from build123d import *

# Parameters (mm, degrees)
SKETCH1_W                                   = 37
SKETCH1_H                                   = 61
BASE_EXTRUSION_DEPTH                        = 1.5875
M2_CLEARANCE_HOLE3_D                        = 2.2
SKETCH8_W                                   = 0.5
SKETCH8_H                                   = 2.2
SIDE_SLOTS_DEPTH                            = 36.707424386
CORNER_BOSS_CLEARANCE_DEPTH                 = 36.707424386
CORNER_BOSS_CLEARANCE_MIRROR_2_COPY_1_DEPTH = 36.707424386
SKETCH10_R                                  = 1.1
AC_WIRE_HOLES_DEPTH                         = 36.707424386


with BuildPart() as part:
    # Sketch1 → Base Extrusion (new body)
    with BuildSketch(Plane(origin=(0, 0, 0), x_dir=(1, 0, 0), z_dir=(0, 1, 0))):
        Rectangle(SKETCH1_W, SKETCH1_H)
    extrude(amount=BASE_EXTRUSION_DEPTH)

    # M2 Clearance Hole3 (through all)
    with Locations(Plane(origin=(0, 1.5875, 0), x_dir=(1, 0, 0), z_dir=(0, 1, 0))):
        with Locations((-18, 10), (-18, -10), (18, -10), (18, 10)):
            Hole(M2_CLEARANCE_HOLE3_D / 2)

    # Sketch8 → Side Slots (cut, through all)
    with BuildSketch(Plane(origin=(0, 1.5875, 0), x_dir=(1, 0, 0), z_dir=(0, 1, 0))):
        with Locations((-18.25, 10)):
            Rectangle(SKETCH8_W, SKETCH8_H)
        with Locations((-18.25, -10)):
            Rectangle(SKETCH8_W, SKETCH8_H)
        with Locations((18.25, 10)):
            Rectangle(SKETCH8_W, SKETCH8_H)
        with Locations((18.25, -10)):
            Rectangle(SKETCH8_W, SKETCH8_H)
    extrude(amount=-SIDE_SLOTS_DEPTH, mode=Mode.SUBTRACT)

    # Sketch9 → Corner Boss Clearance (cut, through all)
    with BuildSketch(Plane(origin=(0, 1.5875, 0), x_dir=(1, 0, 0), z_dir=(0, 1, 0))):
        with BuildLine():
            Line((-18.5, -32.8), (-10.5, -32.8))
            Line((-10.5, -32.8), (-10.5, -28.8))
            ThreePointArc((-10.5, -28.8), (-11.671572875, -25.971572875), (-14.5, -24.8))
            Line((-14.5, -24.8), (-18.5, -24.8))
            Line((-18.5, -24.8), (-18.5, -32.8))
        make_face()
    corner_boss_clearance = extrude(amount=-CORNER_BOSS_CLEARANCE_DEPTH, mode=Mode.SUBTRACT)

    # Corner Boss Clearance Mirror: Corner Boss Clearance across plane
    add(corner_boss_clearance.mirror(Plane(origin=(0, 0, 0), x_dir=(0, 0, 1), z_dir=(1, 0, 0))), mode=Mode.SUBTRACT)

    # Corner Boss Clearance Mirror 2: Corner Boss Clearance across plane
    add(corner_boss_clearance.mirror(Plane.XY), mode=Mode.SUBTRACT)

    # Corner Boss Clearance Mirror 2 copy 1 sk → Corner Boss Clearance Mirror 2 copy 1 (cut, through all)
    with BuildSketch(Plane(origin=(0, 1.5875, 0), x_dir=(-1, 0, 0), z_dir=(0, 1, 0))):
        with BuildLine():
            Line((-18.5, -32.8), (-10.5, -32.8))
            Line((-10.5, -32.8), (-10.5, -28.8))
            ThreePointArc((-10.5, -28.8), (-11.671572875, -25.971572875), (-14.5, -24.8))
            Line((-14.5, -24.8), (-18.5, -24.8))
            Line((-18.5, -24.8), (-18.5, -32.8))
        make_face()
    extrude(amount=-CORNER_BOSS_CLEARANCE_MIRROR_2_COPY_1_DEPTH, mode=Mode.SUBTRACT)

    # Sketch10 → AC Wire Holes (cut, through all)
    with BuildSketch(Plane.XZ):
        with Locations(Location((-5, -27.4, 0), (0, 0, 270))):
            Circle(SKETCH10_R)
        with Locations(Location((5, -27.4, 0), (0, 0, 270))):
            Circle(SKETCH10_R)
        with Locations(Location((-15.4, 17.95, 0), (0, 0, 270))):
            Circle(SKETCH10_R)
        with Locations(Location((-15.4, 2.05, 0), (0, 0, 270))):
            Circle(SKETCH10_R)
    extrude(amount=-AC_WIRE_HOLES_DEPTH, mode=Mode.SUBTRACT)


solid = part.part
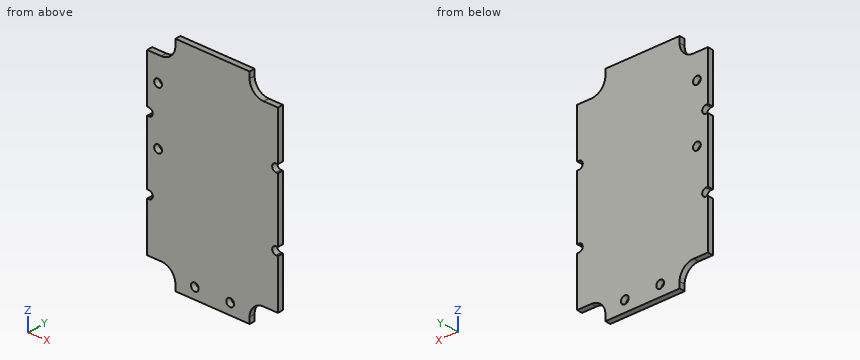
Geometry check sheet. Reference: the model listing, model coordinates, mm. Round coordinates to 2 decimals unless told otherwise and drop trailing zeros. Loops run counter-clockwise (first coordinate to the right, second up) from the corner with the lowest first, then second, coordinate; pieces in that order, holes last. Notation, with made-up numbers: (-14, 43.5) -> (35, 43.5) arc R33 cw to (35, 75.5) -> close; hole circle Ø6 at (67.5, 54). An arc over 180 degrees is marked (long way). Answer as a JSON object with one key per item and string values. Group by question number.
Item 1: Depth check by flat-ended pin: pin 1 Ø0.8 at (y, z) = (1, -30) entering from +X; pin 2 Ø0.5 at (y, z) = (0.5, -29.5) entering from -X. Enter the tip coordinate at first touch or a pass-through.
Item 2: Cross-section at A-A, the plane x = -15.4. Record the cut outline in (y, z).
Item 3: Thickness scan on line 1 along X through (y, z) = (0.5, -27.4); line 2 along X through (y, z) = (0.55, 2.05); line 3 along Z through (x, y) = (-5.5, 0.55). Record the ranges inside material, lowest first.
Item 4: Cross-section at C-C, the plane x = 5. Record the cut outline in (y, z), plus the area to 3 significant figures.
Item 5: Cross-section at B-B, the plane z = 17.95. Record the cut outline in (x, y).
Item 6: Cross-section at D-D, the plane z = -27.4. Record the cut outline in (x, y), plus the area to 3 significant figures.
Determined:
{
 "1": {"pin 1": "stops at x = 10.5", "pin 2": "stops at x = -10.5"},
 "2": {"outline": "(0, -24.8) -> (1.59, -24.8) -> (1.59, 0.95) -> (0, 0.95) -> close; (0, 3.15) -> (1.59, 3.15) -> (1.59, 16.85) -> (0, 16.85) -> close; (0, 19.05) -> (1.59, 19.05) -> (1.59, 24.8) -> (0, 24.8) -> close"},
 "3": {"line 1": "x = -10.75 to -6.1, -3.9 to 3.9, 6.1 to 10.75", "line 2": "x = -18.5 to -16.5, -14.3 to 18.5", "line 3": "z = -30.5 to -28.38, -26.42 to 30.5"},
 "4": {"outline": "(0, -30.5) -> (1.59, -30.5) -> (1.59, -28.5) -> (0, -28.5) -> close; (0, -26.3) -> (1.59, -26.3) -> (1.59, 30.5) -> (0, 30.5) -> close", "area": "93.3 mm²"},
 "5": {"outline": "(-18.5, 0) -> (-16.5, 0) -> (-16.5, 1.59) -> (-18.5, 1.59) -> close; (-14.3, 0) -> (18.5, 0) -> (18.5, 1.59) -> (-14.3, 1.59) -> close"},
 "6": {"outline": "(-10.75, 0) -> (-6.1, 0) -> (-6.1, 1.59) -> (-10.75, 1.59) -> close; (-3.9, 0) -> (3.9, 0) -> (3.9, 1.59) -> (-3.9, 1.59) -> close; (6.1, 0) -> (10.75, 0) -> (10.75, 1.59) -> (6.1, 1.59) -> close", "area": "27.2 mm²"}
}
